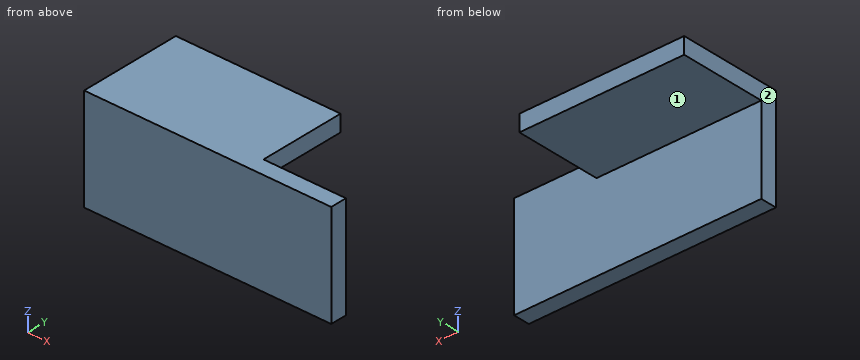
from build123d import *

# Parameters (mm, degrees)
EXTRUDE_1_DEPTH     = 60
SKETCH_2_W          = 20
SKETCH_2_H          = 21
CUT_EXTRUDE_1_DEPTH = 26


with BuildPart() as part:
    # Эскиз1 → Вытянуть-Тонкостенный1 (new body)
    with BuildSketch(Plane(origin=(0, 0, 0), x_dir=(0, 0, -1), z_dir=(1, 0, 0))):
        Polygon((0, 25), (0, 0), (25, 0), (25, 4), (4, 4), (4, 25), align=None)
    extrude(amount=EXTRUDE_1_DEPTH)

    # Эскиз2 → Вырез-Вытянуть1 (cut, through all)
    with BuildSketch(Plane.XY):
        with Locations((50, 14.5)):
            Rectangle(SKETCH_2_W, SKETCH_2_H)
    extrude(amount=-CUT_EXTRUDE_1_DEPTH, mode=Mode.SUBTRACT)


solid = part.part
Design review of the part built by this model. Coordinates are the model's own, in mm. Face numbers are marked on the shaded views. A direction names the side the tool comes from. Round coordinates to 2 decimals unless told otherwise and drop trailing zeros. Write each loop counter-clockwise with the first axis right and the second up, starting at its lowest first coordinate (ties: lowest second). Pieces come first, ordered by that corner, then holes.
Item 1: Consider section C-C on y = 12.5. Give the boundary of the cut face in (x, z).
Item 2: Consider section D-D on x = 46.5. Give the boundary of the cut face in (y, z).
Item 3: Consider section B-B on z = -2.25. Give the boundary of the cut face in (x, y).
Item 4: For pin 1 Ø10.5 at (x, y) = (19.5, 16) entering from -Z; pin 2 Ø3 at (y, z) = (16, -2) entering from +X; pin 3 Ø1 at (x, z) = (19, -15.5) entering from +Y, all flat-tipped, find the tip position at first contact; note any pin that passes through.
Item 5: Consider section A-A on x = 30. Give the boundary of the cut face in (y, z), and give its area (3 significant figures).
Item 6: Wall thickness on L1, parallel to Y at x = 4.5, z = -14; L2, parallel to Z at x = 10, y = 4.5: over which ranges is each line inside the solid? List them lowest first.
Item 7: For the marked faces 1 and 2, list the 3-axis set-ups (+Z, -Z, +X, -X, +Y, -Y) from which the entire face can be reached by the end or side of a thin tool; tool diameter is ignored.
Check values:
1. outline: (0, -4) - (40, -4) - (40, 0) - (0, 0) - close
2. outline: (0, -25) - (4, -25) - (4, 0) - (0, 0) - close
3. outline: (0, 0) - (60, 0) - (60, 4) - (40, 4) - (40, 25) - (0, 25) - close
4. pin 1: stops at z = -4
4. pin 2: stops at x = 40
4. pin 3: stops at y = 4
5. outline: (0, -25) - (4, -25) - (4, -4) - (25, -4) - (25, 0) - (0, 0) - close
5. area: 184 mm2
6. L1: y = 0 to 4
6. L2: z = -4 to 0
7. face 1: -Z, +X, -X, +Y
7. face 2: +Z, -Z, -X, +Y, -Y
